Read the model definition and answer for the solid it produces. Units are mm, in the model's axes. Face numbers are marked on the shaded views. Coordinates: 2 decimals unless noted, no trailing zeros. Write each loop counter-clockwise with the first axis right and the second up, starting at its lowest first coordinate (ties: lowest second). Pieces come first, ordered by that corner, then holes.
(1) Section B-B on y = 0 is taken. Write down the section's boundary in (x, z), then the cut area to 3 significant figures.
(2) The mould has two halves that part along X. Classify the marked faces 1 and 2: +X half, -X half, draft (parallel to the pull), parting line (faces both ways), or undercut.
(3) Given pin 1 (2 mm diameter, centred on x = 16.5, y = 2, fed in from +Z); pin 2 (2.5 mm diameter, centred on y = 18, z = 1.5, fed in from -X); pin 3 (2 mm diameter, centred on x = -19.5, z = 2, fed in from -Y), each flat-ended and moving along its own axis, determine where each tip first touches the part or whether it passes through.
(4) Find the intervals of material crossed by probe 1 along Y at (x, z) = (0, 0.8); probe 2 along Y at (x, z) = (0.5, 2.4); probe 3 along Y at (x, z) = (-8.5, 2.4), in increasing order.
(5) Section A-A on z = 1.9 is taken. State how many separate pieces and enclosed holes the cut face has, then the cut area to 3 significant figures.
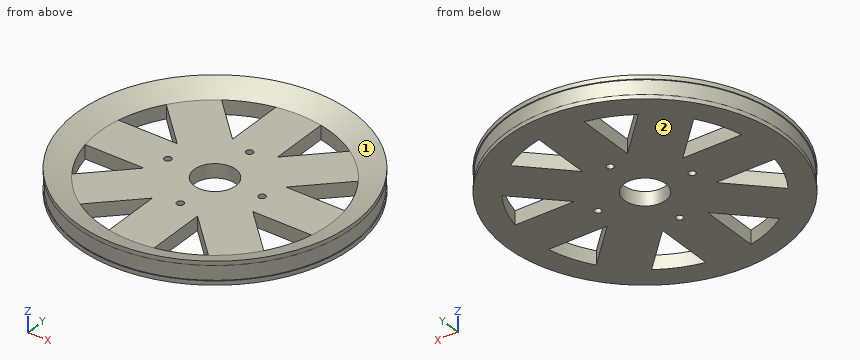
from build123d import *

# Parameters (mm, degrees)
F0_R     = 30
F1_DEPTH = 3
F2_R     = 4.5
F2_R_2   = 0.75
F3_DEPTH = 25
F6_W     = 0.2
F6_H     = 3.2


with BuildPart() as f1:
    # F0 (on Top) → F1 (new body)
    with BuildSketch(Plane.XY):
        Circle(F0_R)
    extrude(amount=F1_DEPTH)

    # F2 (on face) → F3 (cut)
    with BuildSketch(Plane.XY.offset(3)):
        Circle(F2_R)
        with Locations((-10.2, 0)):
            Circle(F2_R_2)
        with Locations((10.2, 0)):
            Circle(F2_R_2)
        with Locations((0, 10.2)):
            Circle(F2_R_2)
        with Locations((0, -10.2)):
            Circle(F2_R_2)
        with BuildLine():
            Line((-4.877146, 11.774472), (-4.877146, 24.519069))
            ThreePointArc((-4.877146, 24.519069), (-9.566866, 23.096458), (-13.888937, 20.786263))
            Line((-13.888937, 20.786263), (-4.877146, 11.774472))
        make_face()
        with BuildLine():
            ThreePointArc((13.888937, 20.786263), (9.566866, 23.096458), (4.877146, 24.519069))
            Line((4.877146, 24.519069), (4.877146, 11.774472))
            Line((4.877146, 11.774472), (13.888937, 20.786263))
        make_face()
        with BuildLine():
            ThreePointArc((-20.786263, 13.888937), (-23.096458, 9.566866), (-24.519069, 4.877146))
            Line((-24.519069, 4.877146), (-11.774472, 4.877146))
            Line((-11.774472, 4.877146), (-20.786263, 13.888937))
        make_face()
        with BuildLine():
            Line((-11.774472, -4.877146), (-24.519069, -4.877146))
            ThreePointArc((-24.519069, -4.877146), (-23.096458, -9.566866), (-20.786263, -13.888937))
            Line((-20.786263, -13.888937), (-11.774472, -4.877146))
        make_face()
        with BuildLine():
            Line((-4.877146, -11.774472), (-13.888937, -20.786263))
            ThreePointArc((-13.888937, -20.786263), (-9.566866, -23.096458), (-4.877146, -24.519069))
            Line((-4.877146, -24.519069), (-4.877146, -11.774472))
        make_face()
        with BuildLine():
            Line((4.877146, -11.774472), (4.877146, -24.519069))
            ThreePointArc((4.877146, -24.519069), (9.566866, -23.096458), (13.888937, -20.786263))
            Line((13.888937, -20.786263), (4.877146, -11.774472))
        make_face()
        with BuildLine():
            Line((11.774472, -4.877146), (20.786263, -13.888937))
            ThreePointArc((20.786263, -13.888937), (23.096458, -9.566866), (24.519069, -4.877146))
            Line((24.519069, -4.877146), (11.774472, -4.877146))
        make_face()
        with BuildLine():
            Line((11.774472, 4.877146), (24.519069, 4.877146))
            ThreePointArc((24.519069, 4.877146), (23.096458, 9.566866), (20.786263, 13.888937))
            Line((20.786263, 13.888937), (11.774472, 4.877146))
        make_face()
    extrude(amount=-F3_DEPTH, mode=Mode.SUBTRACT)

    # F4 (on Front) → F5 (revolve)
    with BuildSketch(Plane.XZ):
        Polygon((-30, 5), (-30, 3), (-25, 3), align=None)
    revolve(axis=Axis((0, 0, 3), (0, 0, 1)))

    # F6 (on Front) → F7 (revolve, cut)
    with BuildSketch(Plane.XZ):
        with Locations((-29.9, 2.5)):
            Rectangle(F6_W, F6_H)
    revolve(axis=Axis((0, 0, 5), (0, 0, 1)), mode=Mode.SUBTRACT)


solid = f1.part
Response:
1. outline: (-30, 0) - (-10.95, 0) - (-10.95, 3) - (-25, 3) - (-30, 5) - (-30, 4.1) - (-29.8, 4.1) - (-29.8, 0.9) - (-30, 0.9) - close; (-9.45, 0) - (-4.5, 0) - (-4.5, 3) - (-9.45, 3) - close; (4.5, 0) - (9.45, 0) - (9.45, 3) - (4.5, 3) - close; (10.95, 0) - (30, 0) - (30, 0.9) - (29.8, 0.9) - (29.8, 4.1) - (30, 4.1) - (30, 5) - (25, 3) - (10.95, 3) - close
1. area: 153 mm2
2. face 1: undercut
2. face 2: draft
3. pin 1: stops at z = 3
3. pin 2: stops at x = -24.78
3. pin 3: stops at y = -23.36
4. probe 1: y = -30 to -10.95, -9.45 to -4.5, 4.5 to 9.45, 10.95 to 30
4. probe 2: y = -29.8 to -10.76, -9.64 to -4.47, 4.47 to 9.64, 10.76 to 29.8
4. probe 3: y = -28.56 to -23.51, -15.4 to 15.4, 23.51 to 28.56
5. separate pieces: 1
5. enclosed holes: 13
5. area: 2,230 mm2
